Autodesk Inventor part; units mm, degrees
ref_plane "YZ Plane" through (0, 0, 0) normal (1, 0, 0) x (0, 1, 0)
ref_plane "XZ Plane" through (0, 0, 0) normal (0, 1, 0) x (-1, 0, 0)
ref_plane "XY Plane" through (0, 0, 0) normal (0, 0, 1) x (1, 0, 0)
sketch "Sketch1" plane through (0, 0, 0) normal (0, 1, 0) x (-1, 0, 0)
  line L0 (18.7, 33.5) -> (-17.7, 33.5)
  line L1 (-17.7, 33.5) -> (-17.7, -33.5)
  line L2 (-17.7, -33.5) -> (18.7, -33.5)
  line L3 (18.7, -33.5) -> (18.7, 33.5)
  point P0 (0, 0)
  dimension "d0" = 36.4
  dimension "d1" = 67
extrude "Extrusion1" add sketch "Sketch1" along normal blind 5
sketch "Sketch2" plane through (0, 5, 0) normal (0, 1, 0) x (1, 0, 0)
  line L0 (-18.7, -33.5) -> (17.7, -33.5)
  line L1 (17.7, -33.5) -> (12.7, -33.5)
  line L2 (12.7, -33.5) -> (12.7, -12.5)
  line L3 (12.7, -12.5) -> (17.7, -12.5)
  line L4 (17.7, -12.5) -> (17.7, -33.5)
  line L5 (17.7, -33.5) -> (17.7, 33.5)
  line L6 (17.7, 33.5) -> (12.7, 33.5)
  line L7 (12.7, 33.5) -> (12.7, 12.5)
  line L8 (12.7, 12.5) -> (17.7, 12.5)
  line L9 (17.7, 12.5) -> (17.7, 33.5)
  point P0 (0, 0)
  dimension "d4" = 5
  dimension "d5" = 21
  dimension "d6" = 5
  dimension "d7" = 21
extrude "Extrusion2" add sketch "Sketch2" along normal blind 25.4
fillet "Fillet2" radius 2 6 edges at (-0.5, 0, 33.5) (-18.7, 0, 0) (17.7, 15.2, 33.5) (17.7, 15.2, -33.5) (-0.5, 0, -33.5) (17.7, 0, 0)
sketch "Sketch6" plane through (0, 5, 0) normal (0, 1, 0) x (1, 0, 0)
  line L0 (-18.7, -33.5) -> (-18.7, 33.5)
  line L1 (-18.7, 12) -> (-13.7, 12)
  line L2 (-13.7, 12) -> (-13.7, -12)
  line L3 (-13.7, -12) -> (-18.7, -12)
  line L4 (-18.7, -12) -> (-18.7, 12)
  point P0 (0, 0)
  point P1 (-18.7, -12)
  dimension "d26" = 5
  dimension "d27" = 24
extrude "Extrusion6" add sketch "Sketch6" along normal blind 25.4
fillet "Fillet3" radius 2 4 edges at (-18.1142, 0.5858, 32.9142) (-18.7, 3.5, 33.5) (-18.1142, 0.5858, -32.9142) (-18.7, 3.5, -33.5)
sketch "Sketch8" plane through (0, 5, 0) normal (0, 1, 0) x (1, 0, 0)
  circle A0 centre (-0.5, 0) radius 4.325
  circle A1 centre (-0.5, -25.4) radius 4.325
  circle A2 centre (-0.5, 25.4) radius 4.325
  point P0 (0, 0)
  dimension "d37" = 8.65
  dimension "d38" = 8.65
  dimension "d39" = 8.65
extrude "Extrusion8" add sketch "Sketch8" along normal blind 3 contours A1 | A2
chamfer "Chamfer1" distance 1.5 angle 45 2 edges at (-4.825, 8, -25.4) (-4.825, 8, 25.4)
sketch "Sketch9" plane through (-0.5, 8, 0) normal (0, 1, 0) x (1, 0, 0)
  circle A0 centre (0, 0) radius 2.825
  circle A1 centre (0, 0) radius 2
  circle A2 centre (0, 25.4) radius 2.825
  circle A3 centre (0, 25.4) radius 2
  circle A4 centre (0, -25.4) radius 2.825
  circle A5 centre (0, -25.4) radius 2
  point P0 (0.5, 0)
  dimension "d45" = 4
  dimension "d46" = 4
  dimension "d47" = 4
extrude "Extrusion9" cut sketch "Sketch9" against normal blind 20 contours A1 | A3 | A5
sketch "Sketch10" plane through (0, 0, 0) normal (0, -1, 0) x (1, 0, 0)
  circle A0 centre (-0.5, -25.4) radius 2.825
  circle A1 centre (-0.5, -25.4) radius 3
  circle A2 centre (-0.5, 0) radius 4.325
  circle A3 centre (-0.5, 0) radius 3
  circle A4 centre (-0.5, 25.4) radius 2.825
  circle A5 centre (-0.5, 25.4) radius 3
  point P0 (0, 0)
  dimension "d50" = 6
  dimension "d51" = 6
  dimension "d52" = 6
extrude "Extrusion10" cut sketch "Sketch10" against normal blind 2.5 contours A0 | A1 | A4 | A5
sketch "Sketch11" plane through (-18.7, 5, 12) normal (-1, 0, 0) x (0, 0, 1)
  line L0 (21.5, 0) -> (0.5, 0)
  line L1 (-29.5, 29.5575) -> (5.5, 29.5575)
  line L2 (5.5, 29.5575) -> (5.5, 0)
  line L3 (5.5, 0) -> (-29.5, 0)
  line L4 (-29.5, 0) -> (-29.5, 29.5575)
  point P0 (-12, -5)
  dimension "d55" = 35
extrude "Extrusion11" cut sketch "Sketch11" against normal blind 50
sketch "Sketch12" plane through (0, 5, 0) normal (0, 1, 0) x (1, 0, 0)
  line L0 (-18.7, 31.5) -> (-18.7, -31.5)
  line L1 (-18.7, 17.5) -> (-13.7, 17.5)
  line L2 (-13.7, 17.5) -> (-13.7, -17.5)
  line L3 (-13.7, -17.5) -> (-18.7, -17.5)
  line L4 (-18.7, -17.5) -> (-18.7, 17.5)
  point P0 (0, 0)
  dimension "d58" = 5
extrude "Extrusion12" add sketch "Sketch12" along normal blind 12.7
properties part number "bigSpringBedMount"
Could you check a few things on this model? Use its own coordinates, in mm. A direction names the side the tool comes from. Coordinates: 2 decimals unless noted, no trailing zeros. Loops run counter-clockwise (first coordinate to the right, second up) from the corner with the lowest first, then second, coordinate; pieces in that order, holes last.
1) Thinking about a two-plate mould opening in X: for faces 1 (the face through (-1.15, 1.23, 22.47)), 2 (the face through (-16, 11, 17.5)), 3 (the face through (-18.7, 8, 0)), 4 (the face through (-13.7, 11, 0)), which applies, released by +X, released by -X, zero draft, split by the parting line, or undercut?
Reported:
face 1: undercut
face 2: zero draft
face 3: released by -X
face 4: released by +X
2) Please list where these lines run through material, in increasing order: line 1 along X through (y, z) = (6.4, 25.4) (3 decimals); line 2 along Z through (x, y) = (0, 2); line 3 along X through (y, z) = (5.5, -9).
Reported:
line 1: x = -4.825 to -2.5, 1.5 to 3.825, 12.7 to 17.7
line 2: z = -33.5 to -28.36, -22.44 to -1.94, 1.94 to 22.44, 28.36 to 33.5
line 3: x = -18.7 to -13.7
3) Which directions (+Z, -Z, +X, -X, +Y, -Y) give clear straight access to the entire face, cutting with the end or side of a thin tool? Please do faces 5 (the face through (1.3, 8, -24.2)), 6 (the face through (0, 2.5, 23)), 7 (the face through (-18.13, 3.48, -32.9)).
Reported:
face 5: +Z, -Z, -X, +Y
face 6: -Y
face 7: -Z, -X, +Y, -Y
4) Will these pins go through, and if not, where does the flat tip stop? pin 1 Ø4 at (x, y) = (-17, 14) entering from -Z; pin 2 Ø2.5 at (x, z) = (-16, 4.5) entering from +Y; pin 3 Ø8 at (y, z) = (20, -5) entering from +X; pin 4 Ø2 at (x, y) = (-6, 7.5) entering from +Z.
Reported:
pin 1: stops at z = -17.5
pin 2: stops at y = 17.7
pin 3: stops at x = -13.7
pin 4: passes through
5) Imagine slicing it at D-D (x = -9). List the corners of the cut face in (y, z) for me, and give its area (3 significant figures).
Reported:
outline: (0, -31.5) arc R2 ccw to (2, -33.5) - (5, -33.5) - (5, 33.5) - (2, 33.5) arc R2 ccw to (0, 31.5) - close
area: 333 mm2
6) Imagine slicing it at B-B (y = 23.5). List the corners of the cut face in (x, z) for me, and give its area (3 significant figures).
Reported:
outline: (12.7, -33.5) - (15.7, -33.5) arc R2 ccw to (17.7, -31.5) - (17.7, -17.5) - (12.7, -17.5) - close; (12.7, 17.5) - (17.7, 17.5) - (17.7, 31.5) arc R2 ccw to (15.7, 33.5) - (12.7, 33.5) - close
area: 158 mm2
7) Imagine slicing it at A-A (y = 9). List the corners of the cut face in (x, z) for me, and give its area (3 significant figures).
Reported:
outline: (-18.7, -17.5) - (-13.7, -17.5) - (-13.7, 17.5) - (-18.7, 17.5) - close; (12.7, -33.5) - (15.7, -33.5) arc R2 ccw to (17.7, -31.5) - (17.7, -17.5) - (12.7, -17.5) - close; (12.7, 17.5) - (17.7, 17.5) - (17.7, 31.5) arc R2 ccw to (15.7, 33.5) - (12.7, 33.5) - close
area: 333 mm2
8) Imagine slicing it at C-C (z = 25.4). List the corners of the cut face in (x, y) for me (3 decimals).
Reported:
outline: (-18.7, 2) arc R2 ccw to (-16.7, 0) - (-3.5, 0) - (-3.5, 2.5) - (-2.5, 2.5) - (-2.5, 8) - (-3.325, 8) - (-4.825, 6.5) - (-4.825, 5) - (-18.7, 5) - close; (1.5, 2.5) - (2.5, 2.5) - (2.5, 0) - (15.7, 0) arc R2 ccw to (17.7, 2) - (17.7, 30.4) - (12.7, 30.4) - (12.7, 5) - (3.825, 5) - (3.825, 6.5) - (2.325, 8) - (1.5, 8) - close
